Autodesk Inventor part; units mm, degrees
ref_plane "YZ Plane" through (0, 0, 0) normal (1, 0, 0) x (0, 1, 0)
ref_plane "XZ Plane" through (0, 0, 0) normal (0, 1, 0) x (-1, 0, 0)
ref_plane "XY Plane" through (0, 0, 0) normal (0, 0, 1) x (1, 0, 0)
sketch "Sketch1" plane through (0, 0, 0) normal (0, 0, 1) x (1, 0, 0)
  line L0 (-18.6, 0) -> (18.6, 0)
  line L1 (18.6, 0) -> (18.6, 2.9)
  line L2 (18.6, 2.9) -> (-18.6, 2.9)
  line L3 (-18.6, 2.9) -> (-18.6, 0)
  line L4 (-18.6, 0) -> (-20.1, 0)
  line L5 (-20.1, 0) -> (-20.1, 2.15)
  line L6 (-20.1, 2.15) -> (-18.6, 2.15)
  line L7 (-18.6, 2.15) -> (-18.6, 0)
  line L8 (-20.1, 0) -> (-29.4, 0)
  line L9 (-29.4, 0) -> (-29.4, 1.55)
  line L10 (-29.4, 1.55) -> (-20.1, 1.55)
  line L11 (-20.1, 1.55) -> (-20.1, 0)
  line L12 (18.6, 0) -> (20.2, 0)
  line L13 (20.2, 0) -> (20.2, 2)
  line L14 (20.2, 2) -> (18.6, 2)
  line L15 (18.6, 2) -> (18.6, 0)
  line L16 (20.2, 0) -> (27.9, 0)
  line L17 (27.9, 0) -> (27.9, 1.5)
  line L18 (27.9, 1.5) -> (20.2, 1.5)
  line L19 (20.2, 1.5) -> (20.2, 0)
  line L20 (27.9, 0) -> (32.9, 0)
  line L21 (32.9, 0) -> (32.9, 1.25)
  line L22 (32.9, 1.25) -> (27.9, 1.25)
  line L23 (27.9, 1.25) -> (27.9, 0)
  point P0 (0, 0)
  point P1 (0, 0)
  dimension "d0" = 9.3
  dimension "d1" = 10.8
  dimension "d2" = 48
  dimension "d3" = 3.1
  dimension "d4" = 4.3
  dimension "d5" = 5.8
  dimension "d6" = 3
  dimension "d7" = 49.6
  dimension "d26" = 2.5
  dimension "d27" = 5
  dimension "d28" = 62.3
  dimension "d29" = 4
revolve "Revolution1" add sketch "Sketch1" angle 360 about axis through (-18.6, 0, 0) along (1, 0, 0)
thread "Thread1"
hole "Hole1" at (-29.4, 0, 0) direction (1, 0, 0) diameter 1.567 depth 6 tip angle 118 counterbore diameter 1.9 counterbore depth 2
sketch "Sketch2" plane through (-29.4, 0, 0) normal (-1, 0, 0) x (0, 0, 1)
  circle A0 centre (0, 0) radius 2.9
  line L0 (-0.8, 2.7875) -> (0.8, 2.7875)
  line L1 (0.8, 2.7875) -> (0.8, 1.4)
  line L2 (0.8, 1.4) -> (-0.8, 1.4)
  line L3 (-0.8, 1.4) -> (-0.8, 2.7875)
  dimension "d22" = 1.6
  dimension "d25" = 4.3
extrude "Extrusion1" cut sketch "Sketch2" against normal blind 53.23 contours L0 A0 | L1 L2 L3 L0
properties part number "401-01" material "Aluminum-6061"
The listing builds one solid part. Answer for the finished solid, in the listing's coordinates (mm). A direction names the side the tool comes from. Give positions to 0.01 mm unless a question says otherwise; leave off trailing zeros. Order: outer loops, then holes, each group sorted by start corner. A loop starts at its lowest first (then second) coordinate and runs counter-clockwise, first axis right, second up. Notation, with made-up numbers: (-22, -13) - (19, -13) arc R20 ccw to (19, -9) - close; hole circle Ø6 at (-25.75, 89). An arc over 180 degrees is marked (long way). Answer in a Markdown table with one row per item. Add a question column.
Q1. The part is cut by section A-A (x = 28.5). Determine the outline of the cut face in (y, z), then the cut area to 3 significant figures.
Q2. The part is cut by section B-B (x = 11). Determine the outline of the cut face in (y, z), then the cut area to 3 significant figures.
Q3. Find the intervals of material crossed by line 1 along Y through (x, z) = (-26.4, 0); line 2 along Y through (x, z) = (-28.85, 0); line 3 along Z through (x, y) = (-25.05, 0), in increasing order. Write a range as [from, to].
Q4. Given P1, Ø1.1, axis at x = -1.5, y = 2, coming from the +Z side; P2, Ø1.1, axis at x = -9.5, y = 2, coming from the -Z side; P3, Ø1, axis at x = 25, y = -1.5, coming from the -Z side, each flat-ended and moving along its own axis, determine where each tip first touches the part or whether it passes through.
Q5. Which of the six approach directions +Z, -Z, +X, -X, +Y, -Y give full straight-line access (tool end or side, diameter ignored) to faces 1 (the flat face through (-20.1, -1.5, 1)), 2 (the flat face through (-3, 1.4, 0)), 3 (the flat face through (20.2, -1.4, 0.9))?
Q6. For a pull along Y with two mould halves and no side action, classify faces 4 (the cylindrical face through (-28.39, -0.04, -0.95)), 5 (the cylindrical face through (-19.34, -2.15, 0.08)), 6 (the flat face through (0, 2, -0.8)) as released by +Y, released by -Y, zero draft, split by the parting line, or undercut.
Determined:
| question | item | result |
|---|---|---|
| 1 | outline | circle Ø2.5 at (0, 0) |
| 1 | area | 4.91 mm² |
| 2 | outline | (1.4, -0.8) - (1.4, 0.8) - (2.79, 0.8) arc R2.9 ccw (long way) to (2.79, -0.8) - close |
| 2 | area | 24.1 mm² |
| 3 | line 1 | y = [-1.55, -0.78], [0.78, 1.4] |
| 3 | line 2 | y = [-1.55, -0.95], [0.95, 1.4] |
| 3 | line 3 | z = [-1.55, -0.78], [0.78, 1.55] |
| 4 | P1 | stops at z = 2.51 |
| 4 | P2 | stops at z = -2.51 |
| 4 | P3 | stops at z = -1.12 |
| 5 | face 1 | -X |
| 5 | face 2 | -X, +Y |
| 5 | face 3 | +X |
| 6 | face 4 | undercut |
| 6 | face 5 | split by the parting line |
| 6 | face 6 | zero draft |
